CAD build for the part. Positions are in the model's coordinates, mm. A direction names the side the tool comes from. Coordinates: 2 decimals unless noted, no trailing zeros. Order: outer loops, then holes, each group sorted by start corner. A loop starts at its lowest first (then second) coordinate and runs counter-clockwise, first axis right, second up. Notation, with made-up numbers: M -19,10 L -5,10 A27 cw -5,49 Z; hole C -35.75,89.25 d6. An arc over 180 degrees is marked long. Write item = value, one per line.
from build123d import *

# Parameters (mm, degrees)
CHAMFER1_R      = 0.5
SKETCH2_R       = 1.07
HOLE_DEPTH      = 6
HOLE_DEPTH_BACK = 6.0000001


with BuildPart() as part:
    # Sketch1 → BaseBody (revolve)
    with BuildSketch(Plane.XY):
        with BuildLine():
            Line((47, 0), (0, 0))
            Line((0, 0), (0, 4))
            ThreePointArc((0, 4), (1, 5), (2, 4))
            Line((2, 4), (2, 3))
            Line((2, 3), (46, 3))
            Line((46, 3), (47, 2.422649731))
            Line((47, 2.422649731), (47, 0))
        make_face()
    revolve(axis=Axis((-19.830028721, 0, 0), (1, 0, 0)))

    # Chamfer1
    chamfer1_edges = [part.edges().sort_by_distance(p)[0] for p in [
        (2, -3, 0),
    ]]
    fillet(chamfer1_edges, radius=CHAMFER1_R)

    # Sketch2 → Hole (cut, two sides)
    with BuildSketch(Plane(origin=(0, 0, 0), x_dir=(1, 0, 0), z_dir=(0, 1, 0))) as hole_sk:
        with Locations((44, 0)):
            Circle(SKETCH2_R)
    extrude(amount=HOLE_DEPTH, mode=Mode.SUBTRACT)
    extrude(hole_sk.sketch, amount=-HOLE_DEPTH_BACK, mode=Mode.SUBTRACT)


solid = part.part
(1) Tool access for faces 1 (the face through (24.55, -0.65, -2.93)), 2 (the face through (0, 0, 0)): list every direction of +Z, -Z, +X, -X, +Y, -Y with a clear straight run to the whole face (end or side of a thin tool).
Evaluation:
face_1 = +X
face_2 = +Z, -Z, -X, +Y, -Y
(2) Slice it at C-C, the plane x = 12. Write the cut outline in (y, z), then the cut area to 3 significant figures.
Evaluation:
outline = C 0,0 d6
area = 28.3 mm²
(3) Pin check, flat tips, straight feed: pin 1 Ø5 at (x, z) = (38, -2) entering from +Y; pin 2 Ø5 at (x, z) = (6, -3) entering from -Y; pin 3 Ø2 at (x, y) = (33, -3) entering from -Z; pin 4 Ø1.5 at (y, z) = (-1, 1) entering from -X. Stop position of each tip, or through.
Evaluation:
pin_1 = 3
pin_2 = -2.96
pin_3 = -2.24
pin_4 = 0
(4) Wall check: line 1 (X direction, y = -0.6, z = 0); line 2 (Z direction, x = 44, y = 1.65); line 3 (Z direction, x = 44, y = -2.4). Give the ranges that are in metal, low to high. Write a range as from..to.
Evaluation:
line_1 = 0..42.93, 45.07..47
line_2 = -2.51..-1.07, 1.07..2.51
line_3 = -1.8..-1.07, 1.07..1.8
(5) Slice it at B-B, the plane x = 44. Write the cut outline in (y, z).
Evaluation:
outline = M -2.8,-1.07 A3 ccw 2.8,-1.07 Z; M -2.8,1.07 L 2.8,1.07 A3 ccw Z
(6) Slice it at A-A, the plane z = 0. Write the cut outline in (x, y).
Evaluation:
outline = M 0,-4 A1 ccw 2,-4 L 2,-3.5 A0.5 cw 2.5,-3 L 42.93,-3 L 42.93,3 L 2.5,3 A0.5 cw 2,3.5 L 2,4 A1 ccw 0,4 Z; M 45.07,-3 L 46,-3 L 47,-2.42 L 47,2.42 L 46,3 L 45.07,3 Z
